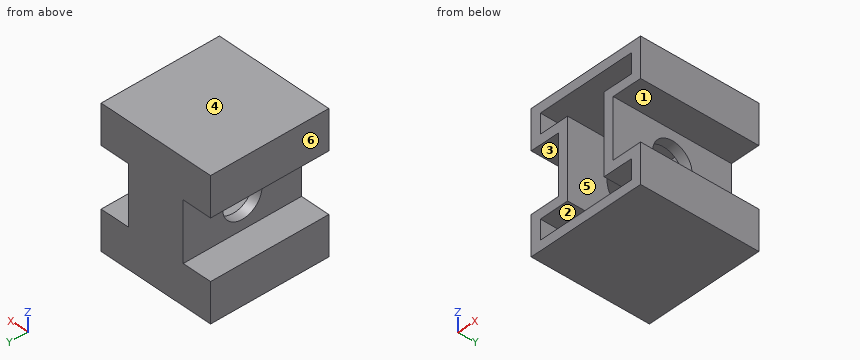
from build123d import *

# Parameters (mm, degrees)
F1_DEPTH = 76.2
F2_T     = -6.35
F3_R     = 12.7
F4_DEPTH = 57.151


with BuildPart() as f1:
    # F0 (on Front) → F1 (new body)
    with BuildSketch(Plane.XZ):
        Polygon((-38.3005267888, -14.7052646339), (-38.3005267888, -40.1052646339), (37.8994732112, -40.1052646339), (37.8994732112, -14.7052646339), (18.8494732112, -14.7052646339), (18.8494732112, 23.3947353661), (37.8994732112, 23.3947353661), (37.8994732112, 48.7947353661), (-38.3005267888, 48.7947353661), (-38.3005267888, 23.3947353661), (-19.2505267888, 23.3947353661), (-19.2505267888, -14.7052646339), align=None)
    extrude(amount=F1_DEPTH)

    # F2
    f2_openings = [f1.faces().sort_by_distance(p)[0] for p in [
        (-0.200527, -76.2, 4.344735),
    ]]
    offset(amount=F2_T, openings=f2_openings, kind=Kind.INTERSECTION)

    # F3 (on face) → F4 (cut, through all)
    with BuildSketch(Plane.YZ.offset(18.8494732112)):
        with Locations((-38.1, 4.3447353661)):
            Circle(F3_R)
    extrude(amount=-F4_DEPTH, mode=Mode.SUBTRACT)


solid = f1.part
For this review, take the finished solid that the model builds, in its own axes (mm). Face numbers are marked on the shaded views. A direction names the side the tool comes from. Round coordinates to 2 decimals unless told otherwise and drop trailing zeros. Order: outer loops, then holes, each group sorted by start corner. A loop starts at its lowest first (then second) coordinate and runs counter-clockwise, first axis right, second up. Notation, with made-up numbers: (39, -12) -> (73, -12) arc R16 ccw to (73, 9) -> close; hole circle Ø4 at (-24, -3.5). An arc over 180 degrees is marked (long way). Put each result on its own line as item: value.
Q1. Insertion check: pin 1 Ø19 at (y, z) = (-51.5, -2) entering from +X; pin 2 Ø19 at (x, z) = (-2, 6) entering from -Y; pin 3 Ø15 at (y, z) = (-38.1, 4.34) entering from +X; pin 4 Ø3 at (y, z) = (-15, 2) entering from -X. Each pin has a flat end and moves straight along its axis. Give the tip position at first contact, or say it passes through.
Check result:
pin 1: x = 18.85
pin 2: y = -6.35
pin 3: through
pin 4: x = -19.25
Q2. For probe 1 along Z at (x, y) = (15, -38); probe 2 along Z at (x, y) = (-26.5, -31); probe 3 along X at (y, z) = (-18, 3.5), list the stretches that pass through material, from the lowest coordinate up. Write a range as [from, to].
Check result:
probe 1: [-40.11, -33.76], [-21.06, -8.35], [17.04, 29.74], [42.44, 48.79]
probe 2: [-40.11, -33.76], [-21.06, -14.71], [23.39, 29.74], [42.44, 48.79]
probe 3: [-19.25, -12.9], [12.5, 18.85]
Q3. Add section C-C on z = -26.5. Write out the cut boundary in (x, y).
Check result:
outline: (-38.3, -76.2) -> (-31.95, -76.2) -> (-31.95, -6.35) -> (31.55, -6.35) -> (31.55, -76.2) -> (37.9, -76.2) -> (37.9, 0) -> (-38.3, 0) -> close
Q4. Add section A-A on x = 27.5. Write out the cut boundary in (y, z).
Check result:
outline: (-76.2, -40.11) -> (0, -40.11) -> (0, -14.71) -> (-76.2, -14.71) -> (-76.2, -21.06) -> (-6.35, -21.06) -> (-6.35, -33.76) -> (-76.2, -33.76) -> close; (-76.2, 23.39) -> (0, 23.39) -> (0, 48.79) -> (-76.2, 48.79) -> (-76.2, 42.44) -> (-6.35, 42.44) -> (-6.35, 29.74) -> (-76.2, 29.74) -> close
Q5. Mouldability with a two-part tool opening along Z and no side actions: class the marked faces 4, 5 and 6 as pulls with the +Z half, pulls with the -Z half, needs draft (parallel to the pull), parting line crosses it, or undercut.
Check result:
face 4: pulls with the +Z half
face 5: undercut
face 6: needs draft
Q6. Machinability: for the marked faces 1, 2 and 3, which of the approach directions +Z, -Z, +X, -X, +Y, -Y give a long, thin tool a straight path to every point of the face, cutting with its end or side? Answer none if there is none.
Check result:
face 1: +X, +Y, -Y
face 2: -Y
face 3: -X, +Y, -Y
Q7. Add section D-D on y = -58.5. Write out the cut boundary in (x, z), plus the area to 3 significant figures.
Check result:
outline: (-38.3, -40.11) -> (37.9, -40.11) -> (37.9, -14.71) -> (18.85, -14.71) -> (18.85, 23.39) -> (37.9, 23.39) -> (37.9, 48.79) -> (-38.3, 48.79) -> (-38.3, 23.39) -> (-19.25, 23.39) -> (-19.25, -14.71) -> (-38.3, -14.71) -> close; hole (-31.95, -33.76) -> (31.55, -33.76) -> (31.55, -21.06) -> (12.5, -21.06) -> (12.5, 29.74) -> (31.55, 29.74) -> (31.55, 42.44) -> (-31.95, 42.44) -> (-31.95, 29.74) -> (-12.9, 29.74) -> (-12.9, -21.06) -> (-31.95, -21.06) -> close
area: 2,420 mm2
